Check sheet for the modelled part. Datum: model origin and axes. Units: mm. Face numbers are marked on the shaded views. Round coordinates to 2 decimals unless told otherwise and drop trailing zeros. Write each loop counter-clockwise with the first axis right and the second up, starting at its lowest first coordinate (ties: lowest second). Pieces come first, ordered by that corner, then holes. Notation, with made-up numbers: (-26.75, 54.25) -> (-8.75, 54.25) arc R21 cw to (-8.75, 84.25) -> close; hole circle Ø11 at (-31, 1). An arc over 180 degrees is marked (long way). Write item = value, one per line.
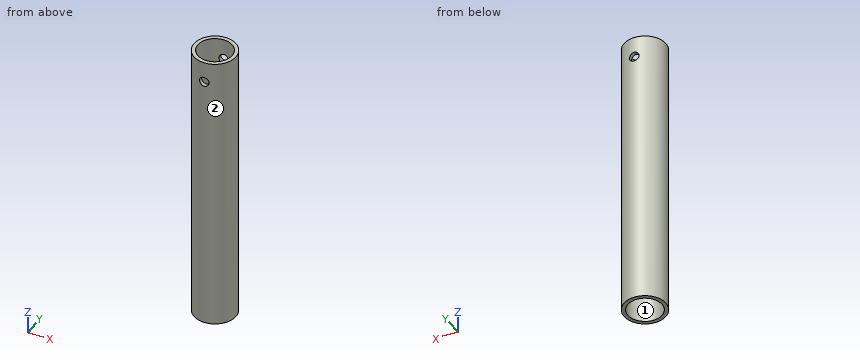
Solid Edge part; units mm, degrees
sketch "Sketch1" plane through (0, 0, 0) normal (0, 0, 1) x (1, 0, 0)
  circle A0 centre (0, 0) radius 11
extrude "Protrusion1" add sketch "Sketch1" along normal mid plane 200
sketch "Sketch2" plane through (0, 0, 100) normal (0, 0, 1) x (1, 0, 0)
  circle A0 centre (0, 0) radius 9
extrude "Cutout1" cut sketch "Sketch2" against normal up to vertex (200 mm away)
sketch "Sketch3" plane through (0, 0, 0) normal (0, -1, 0) x (1, 0, 0)
  circle A0 centre (0, 89) radius 2.5
extrude "ExtrudedCutout_2" cut sketch "Sketch3" along normal mid plane 30
sketch "Sketch4" plane through (0, 0, -100) normal (0, 0, -1) x (1, 0, 0)
  line L0 (-11, 20) -> (19, 20)
  line L1 (19, 20) -> (19.5245, -19.9966)
  line L2 (19.5245, -19.9966) -> (-13.1942, -19.0394)
  line L3 (-13.1942, -19.0394) -> (-11, 20)
extrude "ExtrudedCutout_3" cut sketch "Sketch4" against normal blind 50
(1) Sectioned sample at A-A on x = 0. Enter the section's corners in (y, z).
Worked answers:
outline = (-11, -50) -> (-9, -50) -> (-9, 86.5) -> (-11, 86.5) -> close; (-11, 91.5) -> (-9, 91.5) -> (-9, 100) -> (-11, 100) -> close; (9, -50) -> (11, -50) -> (11, 86.5) -> (9, 86.5) -> close; (9, 91.5) -> (11, 91.5) -> (11, 100) -> (9, 100) -> close
(2) Release check for a two-part mould opening along Y. For the marked faces 1 and 2 record: pulls with the +Y half, pulls with the -Y half, needs draft (parallel to the pull), parting line crosses it, or undercut.
Worked answers:
face_1 = undercut
face_2 = parting line crosses it
(3) Sectioned sample at C-C on z = 89. Enter the section's corners in (x, y), then the cut area to 3 significant figures.
Worked answers:
outline = (-2.5, -10.71) -> (-2.5, -8.65) arc R9 cw to (-2.5, 8.65) -> (-2.5, 10.71) arc R11 ccw to start; (2.5, -10.71) arc R11 ccw to (2.5, 10.71) -> (2.5, 8.65) arc R9 cw to (2.5, -8.65) -> close
area = 105 mm²
(4) Sectioned sample at B-B on y = 0. Enter the section's corners in (x, z), then the cut area to 3 significant figures.
Worked answers:
outline = (-11, -50) -> (-9, -50) -> (-9, 100) -> (-11, 100) -> close; (9, -50) -> (11, -50) -> (11, 100) -> (9, 100) -> close
area = 600 mm²
(5) Material ranges on L1, parallel to Y at x = -0.25, z = 8; L2, parallel to Z at x = 0, y = 9.9; L3, parallel to X at y = -9.7, z = 89, recorded low to high. Write a range as [from, to].
Worked answers:
L1 = [-11, -9], [9, 11]
L2 = [-50, 86.5], [91.5, 100]
L3 = [-5.19, -2.5], [2.5, 5.19]
(6) Go/stop test with flat-tipped pins: P1, Ø3, axis at x = 3, z = 75.5, coming from the -Y side; P2, Ø6, axis at y = 7, z = -29.5, coming from the +X side; P3, Ø10, axis at y = -6, z = 40.5, coming from the +X side. Record where each tip stops, or that it passes through.
Worked answers:
P1 = -10.9
P2 = 10.25
P3 = 10.95
